Read the model definition and answer for the solid it produces. Units are mm, in the model's axes. A direction names the side the tool comes from. Give positions to 0.01 mm unless a question says otherwise; leave off trailing zeros. Order: outer loops, then holes, each group sorted by start corner. A loop starts at its lowest first (then second) coordinate and runs counter-clockwise, first axis right, second up.
```python
from build123d import *

# Parameters (mm, degrees)
F1_DEPTH = 50
F2_W     = 8
F2_H     = 30
F3_DEPTH = 50.001


with BuildPart() as f1:
    # F0 (on Front) → F1 (new body)
    with BuildSketch(Plane.XZ):
        Polygon((0, 20), (0, 0), (80, 0), (80, 50), (60, 50), (60, 20), align=None)
    extrude(amount=-F1_DEPTH)

    # F2 (on Top) → F3 (cut, through all)
    with BuildSketch(Plane.XY):
        with Locations((76, 25)):
            Rectangle(F2_W, F2_H)
    extrude(amount=F3_DEPTH, mode=Mode.SUBTRACT)


solid = f1.part
```
1) The part is cut by section A-A on z = 11. Determine the outline of the cut face in (x, y).
Final values:
outline: (0, 0) - (80, 0) - (80, 10) - (72, 10) - (72, 40) - (80, 40) - (80, 50) - (0, 50) - close
2) For a pull along Y with two mould halves and no side action, classify faces 1 (the face through (48, 0, 14)), 2 (the face through (76, 10, 25)), 3 (the face through (80, 5, 25)) as released by +Y, released by -Y, zero draft, split by the parting line, or undercut.
Final values:
face 1: released by -Y
face 2: undercut
face 3: zero draft
3) The part is cut by section B-B on y = 35.5. Determine the outline of the cut face in (x, z).
Final values:
outline: (0, 0) - (72, 0) - (72, 50) - (60, 50) - (60, 20) - (0, 20) - close
4) Consider L1, parallel to X at y = 23, z = 11; L2, parallel to Z at x = 11.5, y = 47; L3, parallel to X at y = 8, z = 24. Determine where each line is inside the solid, lowest interval first.
Final values:
L1: x = 0 to 72
L2: z = 0 to 20
L3: x = 60 to 80
5) The part is cut by section D-D on z = 21. Determine the outline of the cut face in (x, y), and give its area (3 significant figures).
Final values:
outline: (60, 0) - (80, 0) - (80, 10) - (72, 10) - (72, 40) - (80, 40) - (80, 50) - (60, 50) - close
area: 760 mm2
6) Given pin 1 (3 mm diameter, centred on y = 25, z = 18.5, fed in from +X); pin 2 (4 mm diameter, centred on x = 53.5, y = 33, fed in from +Z), each flat-ended and moving along its own axis, determine where each tip first touches the part or whether it passes through.
Final values:
pin 1: stops at x = 72
pin 2: stops at z = 20
7) The part is cut by section C-C on x = 25.5. Determine the outline of the cut face in (y, z).
Final values:
outline: (0, 0) - (50, 0) - (50, 20) - (0, 20) - close
8) A tool of negligible diameter and unlimited length cuts with its end or side. For faces 4 (the face through (30, 25, 20)), 5 (the face through (80, 45, 25)), 6 (the face through (72, 25, 25)), from which of +Z, -Z, +X, -X, +Y, -Y can it reach the whole face along a straight path? Write none if from no direction.
Final values:
face 4: +Z, -X, +Y, -Y
face 5: +Z, -Z, +X, +Y, -Y
face 6: +Z, -Z, +X
